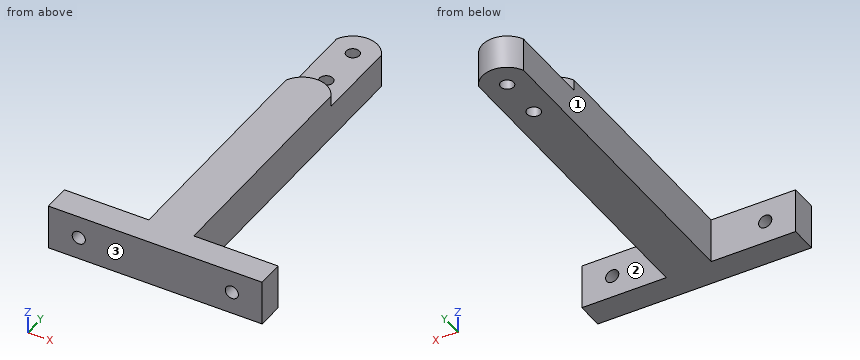
from build123d import *

# Parameters (mm, degrees)
SKETCH1_R           = 3
SKETCH1_R_2         = 2.925
BOSS_EXTRUDE1_DEPTH = 20
CUT_EXTRUDE1_DEPTH  = 5
SKETCH3_R           = 2.925
CUT_EXTRUDE2_DEPTH  = 13


with BuildPart() as part:
    # Sketch1 → Boss-Extrude1 (new body)
    with BuildSketch(Plane.XY):
        with BuildLine():
            Line((-10, -128.247424305), (-10, -269.247424305))
            Line((-10, -269.247424305), (-47.5, -269.247424305))
            Line((-47.5, -269.247424305), (-47.5, -281.247424305))
            Line((-47.5, -281.247424305), (47.5, -281.247424305))
            Line((47.5, -281.247424305), (47.5, -269.247424305))
            Line((47.5, -269.247424305), (10, -269.247424305))
            Line((10, -269.247424305), (10, -128.247424305))
            ThreePointArc((10, -128.247424305), (0, -121.83), (-10, -128.247424305))
        make_face()
        with Locations((0, -152.83)):
            Circle(SKETCH1_R, mode=Mode.SUBTRACT)
        with Locations((0, -132.83)):
            Circle(SKETCH1_R_2, mode=Mode.SUBTRACT)
    extrude(amount=BOSS_EXTRUDE1_DEPTH)

    # Sketch2 → Cut-Extrude1 (cut)
    with BuildSketch(Plane.XY.offset(20)):
        with BuildLine():
            Line((-10, -128.247424305), (-10, -166.247424305))
            ThreePointArc((-10, -166.247424305), (0, -159.83), (10, -166.247424305))
            Line((10, -166.247424305), (10, -128.247424305))
            ThreePointArc((10, -128.247424305), (0, -121.83), (-10, -128.247424305))
        make_face()
    extrude(amount=-CUT_EXTRUDE1_DEPTH, mode=Mode.SUBTRACT)

    # Sketch3 → Cut-Extrude2 (cut, through all)
    with BuildSketch(Plane(origin=(0, -269.247424305, 0), x_dir=(1, 0, 0), z_dir=(0, 1, 0))):
        with Locations((-34, -10)):
            Circle(SKETCH3_R)
        with Locations((34, -10)):
            Circle(SKETCH3_R)
    extrude(amount=-CUT_EXTRUDE2_DEPTH, mode=Mode.SUBTRACT)


solid = part.part
The listing builds one solid part. Answer for the finished solid, in the listing's coordinates (mm). Face numbers are marked on the shaded views. A direction names the side the tool comes from. Give positions to 0.01 mm unless a question says otherwise; leave off trailing zeros. Write each loop counter-clockwise with the first axis right and the second up, starting at its lowest first coordinate (ties: lowest second). Pieces come first, ordered by that corner, then holes. Notation, with made-up numbers: (-11, 73) - (14, 73) arc R6 cw to (14, 78) - close; hole circle Ø1 at (2, -8). An arc over 180 degrees is marked (long way). Use a Markdown table: item, result.
1. Section B-B on y = -132.83 is taken. Write down the section's boundary in (x, z) (3 decimals), plus the area to 3 significant figures.
Values follow:
| item | result |
|---|---|
| outline | (-10, 0) - (-2.925, 0) - (-2.925, 15) - (-10, 15) - close; (2.925, 0) - (10, 0) - (10, 15) - (2.925, 15) - close |
| area | 212 mm² |
2. Section D-D on x = 34 is taken. Write down the section's boundary in (y, z) (3 decimals).
Values follow:
| item | result |
|---|---|
| outline | (-281.247, 0) - (-269.247, 0) - (-269.247, 7.075) - (-281.247, 7.075) - close; (-281.247, 12.925) - (-269.247, 12.925) - (-269.247, 20) - (-281.247, 20) - close |
3. A tool of negligible diameter and unlimited length cuts with its end or side. For the marked faces 1, 2 and 3, from which of +Z, -Z, +X, -X, +Y, -Y can it reach the whole face along a straight path? Write none if from no direction.
Values follow:
| item | result |
|---|---|
| face 1 | +Z, -Z, -X, +Y |
| face 2 | +Z, -Z, +X, +Y |
| face 3 | +Z, -Z, +X, -X, -Y |
4. Each of these flat-tipped pins is pushed along its axis until it touches: P1, Ø1, axis at y = -148, z = 4.5, coming from the +X side; P2, Ø10, axis at x = 22, z = 9.5, coming from the +Y side; P3, Ø10, axis at y = -189.5, z = 8.5, coming from the -X side. Where does it stop, or does it pass through?
Values follow:
| item | result |
|---|---|
| P1 | stops at x = 10 |
| P2 | stops at y = -269.25 |
| P3 | stops at x = -10 |
5. Section C-C on x = 0 is taken. Write down the section's boundary in (y, z) (3 decimals), plus the area to 3 significant figures.
Values follow:
| item | result |
|---|---|
| outline | (-281.247, 0) - (-155.83, 0) - (-155.83, 15) - (-159.83, 15) - (-159.83, 20) - (-281.247, 20) - close; (-149.83, 0) - (-135.755, 0) - (-135.755, 15) - (-149.83, 15) - close; (-129.905, 0) - (-121.83, 0) - (-121.83, 15) - (-129.905, 15) - close |
| area | 2,820 mm² |
6. Section A-A on z = 10 is taken. Write down the section's boundary in (x, y) (3 decimals), plus the area to 3 significant figures.
Values follow:
| item | result |
|---|---|
| outline | (-47.5, -281.247) - (-36.925, -281.247) - (-36.925, -269.247) - (-47.5, -269.247) - close; (-31.075, -281.247) - (31.075, -281.247) - (31.075, -269.247) - (10, -269.247) - (10, -128.247) arc R11 ccw to (-10, -128.247) - (-10, -269.247) - (-31.075, -269.247) - close; (36.925, -281.247) - (47.5, -281.247) - (47.5, -269.247) - (36.925, -269.247) - close; hole circle Ø6 at (0, -152.83); hole circle Ø5.85 at (0, -132.83) |
| area | 3,860 mm² |
7. Find the intervals of material crossed by probe 1 along X at (y, z) = (-278, 10) (3 decimals); probe 2 along Z at (x, y) = (34, -273.75) (3 decimals); probe 3 along X at (y, z) = (-152.83, 3.75), in increasing order. Write a range as from..to.
Values follow:
| item | result |
|---|---|
| probe 1 | x = -47.5..-36.925, -31.075..31.075, 36.925..47.5 |
| probe 2 | z = 0..7.075, 12.925..20 |
| probe 3 | x = -10..-3, 3..10 |
